from build123d import *

# Parameters (mm, degrees)
F0_W      = 260
F0_H      = 40
F1_DEPTH  = 5
F2_W      = 170
F2_H      = 5
F3_DEPTH  = 35
F5_DEPTH  = 5
F7_DEPTH  = 35
F8_R      = 4
F9_DEPTH  = 25
F10_DEPTH = 25


with BuildPart() as f1:
    # F0 (on Top) → F1 (new body)
    with BuildSketch(Plane.XY):
        Rectangle(F0_W, F0_H)
    extrude(amount=F1_DEPTH)

    # F2 (on face) → F3 (join)
    with BuildSketch(Plane(origin=(0, 0, 0), x_dir=(1, 0, 0), z_dir=(0, 0, -1))):
        with Locations((-5, 17.5)):
            Rectangle(F2_W, F2_H)
    extrude(amount=F3_DEPTH)

    # F4 (on face) → F5 (join)
    with BuildSketch(Plane(origin=(0, 0, 0), x_dir=(1, 0, 0), z_dir=(0, 0, -1))):
        with BuildLine():
            ThreePointArc((-110, 59), (-112.828427, 52.171573), (-106, 55))
            ThreePointArc((-106, 55), (-107.171573, 57.828427), (-110, 59))
        make_face()
        Polygon((-130, 80), (-130, 20), (-90, 20), (-90, 80), (-110, 80), align=None)
        with BuildLine():
            ThreePointArc((-106, 55), (-112.828427, 52.171573), (-110, 59))
            ThreePointArc((-110, 59), (-107.171573, 57.828427), (-106, 55))
        make_face(mode=Mode.SUBTRACT)
    extrude(amount=-F5_DEPTH)

    # F6 (on face) → F7 (join)
    with BuildSketch(Plane(origin=(0, 0, 0), x_dir=(1, 0, 0), z_dir=(0, 0, -1))):
        Polygon((-95, 15), (-90, 15), (-90, 20), (-90, 30), (-95, 30), align=None)
    extrude(amount=F7_DEPTH)

    # F8 (on face) → F9 (cut)
    with BuildSketch(Plane.XY.offset(5)):
        with Locations((-110, -150)):
            Circle(F8_R)
        with Locations((100, 0)):
            Circle(F8_R)
    extrude(amount=-F9_DEPTH, mode=Mode.SUBTRACT)

    # F4 (on face) → F10 (cut)
    with BuildSketch(Plane(origin=(0, 0, 0), x_dir=(1, 0, 0), z_dir=(0, 0, -1))):
        with BuildLine():
            ThreePointArc((-110, 59), (-112.828427, 52.171573), (-106, 55))
            ThreePointArc((-106, 55), (-107.171573, 57.828427), (-110, 59))
        make_face()
    extrude(amount=-F10_DEPTH, mode=Mode.SUBTRACT)


solid = f1.part
Verification items for the finished model (mm, model axes). A direction names the side the tool comes from. Coordinates: 2 decimals unless noted, no trailing zeros. Write each loop counter-clockwise with the first axis right and the second up, starting at its lowest first coordinate (ties: lowest second). Pieces come first, ordered by that corner, then holes. Notation, with made-up numbers: M 69.25,25.25 L 120.25,25.25 A21 ccw 120.25,45.25 Z; hole C 44,59.5 d4. An arc over 180 degrees is marked long. Use a Markdown table: item, result.
Q1. Sectioned sample at B-B, the plane x = 100. Record the boundary of the cut face in (y, z), plus the area to 3 significant figures.
Reply:
| item | result |
|---|---|
| outline | M -20,0 L -4,0 L -4,5 L -20,5 Z; M 4,0 L 20,0 L 20,5 L 4,5 Z |
| area | 160 mm² |
Q2. Sectioned sample at C-C, the plane z = -16. Record the boundary of the cut face in (x, y).
Reply:
| item | result |
|---|---|
| outline | M -95,-30 L -90,-30 L -90,-20 L 80,-20 L 80,-15 L -95,-15 Z |
Q3. Sectioned sample at D-D, the plane y = -44. Record the boundary of the cut face in (x, z), plus the area to 3 significant figures.
Reply:
| item | result |
|---|---|
| outline | M -130,0 L -90,0 L -90,5 L -130,5 Z |
| area | 200 mm² |
Q4. Sectioned sample at A-A, the plane y = 0. Record the boundary of the cut face in (x, z), plus the area to 3 significant figures.
Reply:
| item | result |
|---|---|
| outline | M -130,0 L 96,0 L 96,5 L -130,5 Z; M 104,0 L 130,0 L 130,5 L 104,5 Z |
| area | 1,260 mm² |
Q5. Go/stop test with flat-tipped pins: P1, Ø1.5, axis at x = -91.5, z = -13.5, coming from the -Y side; P2, Ø20, axis at x = 12, z = -20.5, coming from the -Y side; P3, Ø1, axis at y = -22.5, z = -11.5, coming from the -X side; P4, Ø7, axis at x = 100, y = 0, coming from the -Z side. Record where each tip stops, or that it passes through.
Reply:
| item | result |
|---|---|
| P1 | stops at y = -30 |
| P2 | stops at y = -20 |
| P3 | stops at x = -95 |
| P4 | passes through |
Q6. Set-up check for faces 1 (the face through (-92, -30, -17)), 2 (the face through (-95, -23, -17)), 3 (the face through (-90, -28, -12)): record each of +Z, -Z, +X, -X, +Y, -Y from which the full face is reachable in a straight line by a thin tool's end or side.
Reply:
| item | result |
|---|---|
| face 1 | -Z, +X, -X, -Y |
| face 2 | -Z, -X, +Y, -Y |
| face 3 | +Z, -Z, +X, -Y |
Q7. Thickness scan on line 1 (X direction, y = -55, z = 1.6); line 2 (Y direction, x = -110, z = 3.6); line 3 (Y direction, x = 60, z = -2). Record the ranges inside material, lowest first.
Reply:
| item | result |
|---|---|
| line 1 | x = -130 to -114, -106 to -90 |
| line 2 | y = -80 to -59, -51 to 20 |
| line 3 | y = -20 to -15 |
